```python
from build123d import *

# Parameters (mm, degrees)
SKETCH1_W           = 31.87
SKETCH1_H           = 71.6
BOSS_EXTRUDE1_DEPTH = 56.17
SKETCH2_W           = 72.17
SKETCH2_H           = 87.6
SKETCH2_W_2         = 58.17
SKETCH2_H_2         = 73.6
BOSS_EXTRUDE4_DEPTH = 31.87
SKETCH5_W           = 72.17
SKETCH5_H           = 87.6
BOSS_EXTRUDE5_DEPTH = 7
SKETCH6_W           = 24.87
SKETCH6_H           = 71.6
CUT_EXTRUDE2_DEPTH  = 92.222513257
SKETCH7_R           = 7
BOSS_EXTRUDE6_DEPTH = 20
BOSS_EXTRUDE7_START = -20
SKETCH8_R           = 7
BOSS_EXTRUDE7_DEPTH = 20
SKETCH9_R           = 2.753
SKETCH9_R_2         = 2.75
SKETCH9_R_3         = 2.45
CUT_EXTRUDE3_DEPTH  = 20
CUT_EXTRUDE4_DEPTH  = 40
SKETCH11_W          = 18.463529731
SKETCH11_H          = 14.991415607
CUT_EXTRUDE5_DEPTH  = 10
SKETCH12_R          = 2
CUT_EXTRUDE6_DEPTH  = 105.629761182
SKETCH13_W          = 1.5
SKETCH13_H          = 49.254465911
CUT_EXTRUDE7_DEPTH  = 128.892872897
SKETCH14_W          = 12
SKETCH14_H          = 12
BOSS_EXTRUDE8_DEPTH = 12
SKETCH15_R          = 4
CUT_EXTRUDE8_DEPTH  = 12
FILLET1_R           = 1.5


with BuildPart() as part:
    # Sketch1 → Boss-Extrude1 (new body)
    with BuildSketch(Plane(origin=(0, 0, 0), x_dir=(0, 0, -1), z_dir=(1, 0, 0))):
        Rectangle(SKETCH1_W, SKETCH1_H)
    extrude(amount=BOSS_EXTRUDE1_DEPTH)



with BuildPart() as body_2:
    # Sketch2 → Boss-Extrude4 (new body)
    with BuildSketch(Plane(origin=(0, 0, -15.935), x_dir=(-1, 0, 0), z_dir=(0, 0, -1))):
        with Locations((-28.085, 0)):
            Rectangle(SKETCH2_W, SKETCH2_H)
        with Locations((-28.085, 0)):
            Rectangle(SKETCH2_W_2, SKETCH2_H_2, mode=Mode.SUBTRACT)
    extrude(amount=BOSS_EXTRUDE4_DEPTH)


with BuildPart() as part_1:
    add(part.part)

    add(body_2.part)  # Boss-Extrude5 merges body 2
    # Sketch5 → Boss-Extrude5 (add)
    with BuildSketch(Plane.XY.offset(-15.935)):
        with Locations((28.085, 0)):
            Rectangle(SKETCH5_W, SKETCH5_H)
    extrude(amount=BOSS_EXTRUDE5_DEPTH)

    # Sketch6 → Cut-Extrude2 (cut, through all)
    with BuildSketch(Plane.ZY):
        with Locations((3.5, 0)):
            Rectangle(SKETCH6_W, SKETCH6_H)
    extrude(amount=-CUT_EXTRUDE2_DEPTH, mode=Mode.SUBTRACT)

    # Sketch7 → Boss-Extrude6 (add)
    with BuildSketch(Plane.ZY.offset(8)):
        with Locations((-47.805, -45.3)):
            Circle(SKETCH7_R)
    extrude(amount=-BOSS_EXTRUDE6_DEPTH)

    # Sketch8 → Boss-Extrude7 (add)
    with BuildSketch(Plane(origin=(64.17, 0, 0), x_dir=(0, 0, -1), z_dir=(1, 0, 0)).offset(BOSS_EXTRUDE7_START)):
        with Locations((47.805, -45.3)):
            Circle(SKETCH8_R)
    extrude(amount=BOSS_EXTRUDE7_DEPTH)

    # Sketch9 → Cut-Extrude3 (cut)
    with BuildSketch(Plane(origin=(0, 43.8, 0), x_dir=(1, 0, 0), z_dir=(0, 1, 0))):
        with Locations(Location((41.35, 32.555, 0), (0, 0, 270))):
            Circle(SKETCH9_R)
        with Locations(Location((28.65, 32.555, 0), (0, 0, 270))):
            Circle(SKETCH9_R_2)
        with Locations(Location((15.95, 32.555, 0), (0, 0, 270))):
            Circle(SKETCH9_R_3)
    extrude(amount=-CUT_EXTRUDE3_DEPTH, mode=Mode.SUBTRACT)

    # Sketch10 → Cut-Extrude4 (cut)
    with BuildSketch(Plane(origin=(0, 0, -47.805), x_dir=(-1, 0, 0), z_dir=(0, 0, -1))):
        with BuildLine():
            Line((-33.567827079, -43.8), (-21.344405358, -43.8))
            ThreePointArc((-21.344405358, -43.8), (-27.456116219, -39.739220659), (-33.567827079, -43.8))
        make_face()
    extrude(amount=-CUT_EXTRUDE4_DEPTH, mode=Mode.SUBTRACT)

    # Sketch11 → Cut-Extrude5 (cut)
    with BuildSketch(Plane.ZY.offset(8)):
        with Locations((-34.516340539, -19.295707804)):
            Rectangle(SKETCH11_W, SKETCH11_H)
    extrude(amount=-CUT_EXTRUDE5_DEPTH, mode=Mode.SUBTRACT)

    # Sketch12 → Cut-Extrude6 (cut, through all)
    with BuildSketch(Plane.ZY.offset(8)):
        with Locations((-47.805, -45.3)):
            Circle(SKETCH12_R)
    extrude(amount=-CUT_EXTRUDE6_DEPTH, mode=Mode.SUBTRACT)

    # Sketch13 → Cut-Extrude7 (cut, through all)
    with BuildSketch(Plane(origin=(0, 43.8, 0), x_dir=(1, 0, 0), z_dir=(0, 1, 0))):
        with Locations((63.42, 33.562232956)):
            Rectangle(SKETCH13_W, SKETCH13_H)
    extrude(amount=-CUT_EXTRUDE7_DEPTH, mode=Mode.SUBTRACT)

    # Sketch14 → Boss-Extrude8 (add)
    with BuildSketch(Plane.XY.offset(-8.935)):
        with Locations((56.67, 22.541140532)):
            Rectangle(SKETCH14_W, SKETCH14_H)
    extrude(amount=BOSS_EXTRUDE8_DEPTH)

    # Sketch15 → Cut-Extrude8 (cut)
    with BuildSketch(Plane(origin=(62.67, 0, 0), x_dir=(0, 0, -1), z_dir=(1, 0, 0))):
        with Locations((2.935, 28.541140532)):
            Circle(SKETCH15_R)
    extrude(amount=-CUT_EXTRUDE8_DEPTH, mode=Mode.SUBTRACT)

    # Fillet1
    fillet1_edges = [part_1.edges().sort_by_distance(p)[0] for p in [
        (56.67, 28.541140532, -8.935),
        (50.67, 22.541140532, -8.935),
        (56.67, 16.541140532, -8.935),
        (62.67, 22.541140532, 3.065),
        (50.67, 22.541140532, 3.065),
        (56.67, 16.541140532, 3.065),
    ]]
    fillet(fillet1_edges, radius=FILLET1_R)


solid = part_1.part
```
Read the model definition and answer for the solid it produces. Units are mm, in the model's axes. A direction names the side the tool comes from. Give positions to 0.01 mm unless a question says otherwise; leave off trailing zeros. Write each loop counter-clockwise with the first axis right and the second up, starting at its lowest first coordinate (ties: lowest second). Pieces come first, ordered by that corner, then holes. Notation, with made-up numbers: M 39.5,-11 L 73.5,-11 A24 cw 73.5,15 Z; hole C 52,62 d1. An arc over 180 degrees is marked long. Put each result on its own line as item: value. Start each with the question number.
1. Each of these flat-tipped pins is pushed along its axis until it touches: pin 1 Ø4 at (x, y) = (53, -25.5) entering from +Z (3 decimals); pin 2 Ø1.5 at (x, z) = (44.5, -14.5) entering from -Y; pin 3 Ø12 at (x, z) = (39.5, -40) entering from -Y. Where does it stop, or does it pass through?
2. The part is cut by section C-C, the plane z = -23.5. Give the vertices of the cut face in (x, y).
3. The part is cut by section B-B, the plane x = 15.95. Give the vertices of the cut face in (y, z) (3 decimals).
4. Consider line 1 along Y through (x, z) = (20, -28); line 2 along X through (y, z) = (-29.5, -24); line 3 along Y through (x, z) = (6.5, -47.5). Determine where each line is inside the solid, lowest interval first.
5. Which of the six approach directions +Z, -Z, +X, -X, +Y, -Y give full straight-line access (tool end or side, diameter ignored) to faces 1 (the cylindrical face through (14.46, 40.35, -34.5)), 2 (the flat face through (-5, -11.8, -35)), 3 (the flat face through (28, 1, -15.935)), 4 (the cylindrical face through (27.35, -39.74, -28.64)), 5 (the flat face through (57, 23, 3.065))?
6. For a pull along X with two mould halves and no side action, classify faces 6 (the cylindrical face through (53.29, -50.902, -52.002)), 7 (the cylindrical face through (44.08, 40.35, -32.91)) as released by +X, released by -X, zero draft, split by the parting line, or undercut.
7. The part is cut by section D-D, the plane y = -18.5. Give the vertices of the cut face in (x, z) (3 decimals).
8. The part is cut by section A-A, the plane y = -45.3. Give the vertices of the cut face in (x, z) (3 decimals).
Final values:
1. pin 1: stops at z = -8.935
1. pin 2: stops at y = -43.8
1. pin 3: stops at y = -51.02
2. outline: M -8,-43.8 L 21.34,-43.8 A6.63 cw 33.57,-43.8 L 62.67,-43.8 L 62.67,43.8 L -8,43.8 Z; hole M -1,-36.8 L 57.17,-36.8 L 57.17,36.8 L -1,36.8 Z
3. outline: M -43.8,-46.482 A2 cw -43.3,-47.805 L -36.8,-47.805 L -36.8,-15.935 L 36.8,-15.935 L 36.8,-30.105 L 43.8,-30.105 L 43.8,-8.935 L -43.8,-8.935 Z; M 36.8,-47.805 L 43.8,-47.805 L 43.8,-35.005 L 36.8,-35.005 Z
4. line 1: y = -43.8 to -36.8, 36.8 to 43.8
4. line 2: x = -8 to -1, 57.17 to 62.67
4. line 3: y = -52.29 to -47.28, -43.32 to -36.8, 36.8 to 43.8
5. face 1: +Y
5. face 2: -X
5. face 3: -Z
5. face 4: +Z, -Z, -Y
5. face 5: +Z, +X, -X, +Y, -Y
6. face 6: zero draft
6. face 7: undercut
7. outline: M -8,-47.805 L -1,-47.805 L -1,-43.748 L -8,-43.748 Z; M -8,-25.285 L -1,-25.285 L -1,-15.935 L 57.17,-15.935 L 57.17,-47.805 L 62.67,-47.805 L 62.67,-8.935 L -8,-8.935 Z
8. outline: M -8,-54.805 L 12,-54.805 L 12,-49.805 L -8,-49.805 Z; M -8,-45.805 L 12,-45.805 L 12,-40.805 L -8,-40.805 Z; M 44.17,-54.805 L 62.67,-54.805 L 62.67,-49.805 L 44.17,-49.805 Z; M 44.17,-45.805 L 62.67,-45.805 L 62.67,-40.805 L 44.17,-40.805 Z
